Here's how the part is built. I have some questions about the finished solid (model axes, mm). A direction names the side the tool comes from. Give positions to 0.01 mm unless a question says otherwise; leave off trailing zeros. Use a Markdown table: item, result.
```python
from build123d import *

# Parameters (mm, degrees)
SKETCH1_W           = 10.53028371
SKETCH1_H           = 7.9375
BOSS_EXTRUDE1_DEPTH = 6.35
SKETCH2_W           = 10.53028371
SKETCH2_H           = 15.875
BOSS_EXTRUDE2_DEPTH = 11.1125
SKETCH3_R           = 0.75
BOSS_EXTRUDE3_DEPTH = 3.5


with BuildPart() as part:
    # Sketch1 → Boss-Extrude1 (new body)
    with BuildSketch(Plane(origin=(0, 0, 0), x_dir=(1, 0, 0), z_dir=(0, 1, 0))):
        with BuildLine():
            Line((-5.265141855, 0), (-5.265141855, 7.9375))
            ThreePointArc((-5.265141855, 7.9375), (-8.392737967, 4.504173), (-9.525, 0))
            Line((-9.525, 0), (-5.265141855, 0))
        make_face()
        with BuildLine():
            Line((-5.265141855, -7.9375), (-5.265141855, 0))
            Line((-5.265141855, 0), (-9.525, 0))
            ThreePointArc((-9.525, 0), (-8.392737967, -4.504173), (-5.265141855, -7.9375))
        make_face()
        with Locations((0, -3.96875)):
            Rectangle(SKETCH1_W, SKETCH1_H)
        with BuildLine():
            ThreePointArc((9.525, 0), (8.392737967, 4.504173), (5.265141855, 7.9375))
            Line((5.265141855, 7.9375), (5.265141855, 0))
            Line((5.265141855, 0), (9.525, 0))
        make_face()
        with BuildLine():
            Line((9.525, 0), (5.265141855, 0))
            Line((5.265141855, 0), (5.265141855, -7.9375))
            ThreePointArc((5.265141855, -7.9375), (8.392737967, -4.504173), (9.525, 0))
        make_face()
        with BuildLine():
            ThreePointArc((-9.525, 0), (-8.392737967, 4.504173), (-5.265141855, 7.9375))
            ThreePointArc((-5.265141855, 7.9375), (0, 9.525), (5.265141855, 7.9375))
            ThreePointArc((5.265141855, 7.9375), (8.392737967, 4.504173), (9.525, 0))
            Line((9.525, 0), (9.525, 15.875))
            Line((9.525, 15.875), (-9.525, 15.875))
            Line((-9.525, 15.875), (-9.525, 0))
        make_face()
        with Locations((0, 3.96875)):
            Rectangle(SKETCH1_W, SKETCH1_H)
        with BuildLine():
            ThreePointArc((5.265141855, 7.9375), (0, 9.525), (-5.265141855, 7.9375))
            Line((-5.265141855, 7.9375), (5.265141855, 7.9375))
        make_face()
    extrude(amount=BOSS_EXTRUDE1_DEPTH)

    # Sketch2 → Boss-Extrude2 (add)
    with BuildSketch(Plane(origin=(0, 6.35, 0), x_dir=(1, 0, 0), z_dir=(0, 1, 0))):
        with BuildLine():
            Line((-5.265141855, -7.9375), (-5.265141855, 7.9375))
            ThreePointArc((-5.265141855, 7.9375), (-8.392737967, 4.504173), (-9.525, 0))
            ThreePointArc((-9.525, 0), (-8.392737967, -4.504173), (-5.265141855, -7.9375))
        make_face()
        Rectangle(SKETCH2_W, SKETCH2_H)
        with BuildLine():
            ThreePointArc((9.525, 0), (8.392737967, 4.504173), (5.265141855, 7.9375))
            Line((5.265141855, 7.9375), (5.265141855, -7.9375))
            ThreePointArc((5.265141855, -7.9375), (8.392737967, -4.504173), (9.525, 0))
        make_face()
    extrude(amount=BOSS_EXTRUDE2_DEPTH)

    # Sketch3 → Boss-Extrude3 (add)
    with BuildSketch(Plane(origin=(0, 17.4625, 0), x_dir=(1, 0, 0), z_dir=(0, 1, 0))):
        Circle(SKETCH3_R)
    extrude(amount=BOSS_EXTRUDE3_DEPTH)


solid = part.part
```
Item 1: For faces 1 (the flat face through (0, 12, -7.938)), 2 (the cylindrical face through (-0.75, 19.19, -0.03)), 3 (the flat face through (0, 9, 7.938)), which set-ups out of +Z, -Z, +X, -X, +Y, -Y let a thin tool reach every point of the face, with its end or its side?
Values:
| item | result |
|---|---|
| face 1 | -Z, +X, -X, +Y |
| face 2 | +Y |
| face 3 | +Z, +X, -X, +Y, -Y |
Item 2: I need wall thicknesses on line 1 along Y through (x, z) = (0.25, -3); line 2 along Z through (x, y) = (-3.25, 11.5); line 3 along Y through (x, z) = (-8.25, -11.25). Which ranges of each line are inside material? Lowest first, please. Write a range as [from, to].
Values:
| item | result |
|---|---|
| line 1 | y = [0, 17.46] |
| line 2 | z = [-7.94, 7.94] |
| line 3 | y = [0, 6.35] |
Item 3: Will these pins go through, and if not, where does the flat tip stop? pin 1 Ø2 at (y, z) = (7, 4.5) entering from -X; pin 2 Ø3 at (x, y) = (1, 12) entering from -Z; pin 3 Ø5 at (y, z) = (3.5, 2) entering from +X (3 decimals).
Values:
| item | result |
|---|---|
| pin 1 | stops at x = -8.86 |
| pin 2 | stops at z = -7.94 |
| pin 3 | stops at x = 9.525 |
